Can you work these out from the drawing? Everything is in mm from the part's minimum corner. Round coordinates to 2 decimals unless told otherwise and drop trailing zeros. Loops run counter-clockwise (first coordinate to the right, second up) from the corner with the lowest first, then second, coordinate; pieces in that order, holes last. Notation, with made-up numbers: (-25.5, -37.75) -> (20.5, -37.75) arc R23 cw to (20.5, -21.75) -> close; hole circle Ø11 at (43, 46.25). An arc over 180 degrees is marked (long way). One line per item, written item: value.
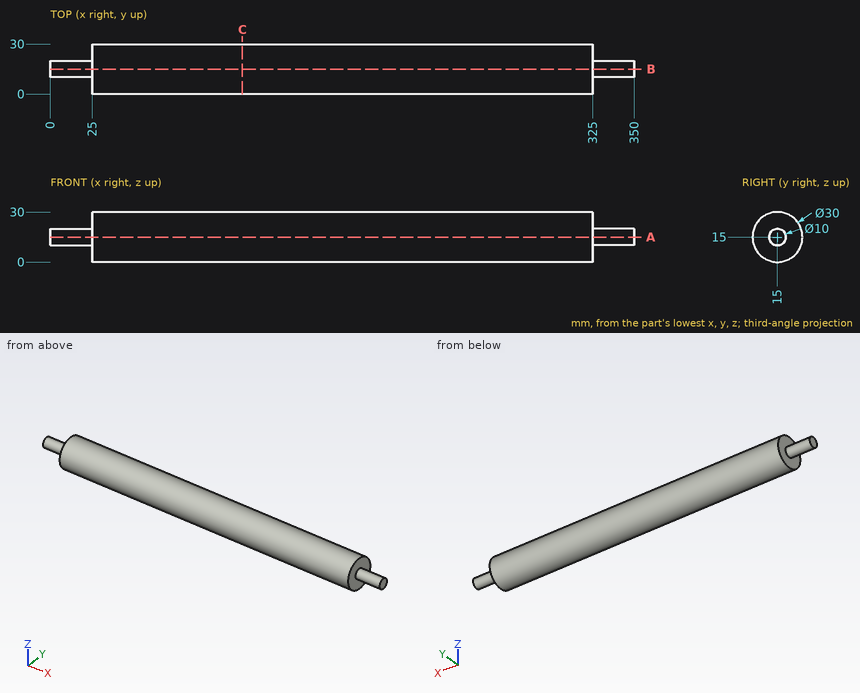
Item 1: Will these pins go through, and if not, where does the flat tip stop? pin 1 Ø1 at (y, z) = (6, 3.5) entering from +X; pin 2 Ø4 at (x, z) = (182.5, 8.5) entering from +Y; pin 3 Ø1.5 at (x, z) = (107, 26.5) entering from +Y.
Output:
pin 1: stops at x = 325
pin 2: stops at y = 29.31
pin 3: stops at y = 25.46
Item 2: I need wall thicknesses on line 1 (X direction, y = 16, z = 2.5); line 2 (Y direction, x = 30.5, z = 15.75); line 3 (Z direction, x = 156.5, y = 13.75). Which ranges of each line are inside material? Lowest first, please. Write a range as from..to.
Output:
line 1: x = 25..325
line 2: y = 0.02..29.98
line 3: z = 0.05..29.95
Item 3: If we section it at A-A on z = 15: List the corners of the cut face in (x, y) for me.
Output:
outline: (0, 10) -> (25, 10) -> (25, 0) -> (325, 0) -> (325, 10) -> (350, 10) -> (350, 20) -> (325, 20) -> (325, 30) -> (25, 30) -> (25, 20) -> (0, 20) -> close
Item 4: If we section it at C-C on x = 115: List the corners of the cut face in (y, z) for me, plus the area to 3 significant figures.
Output:
outline: circle Ø30 at (15, 15)
area: 707 mm²
